Geometry check sheet. Reference: the model listing, model coordinates, mm. A direction names the side the tool comes from. Give positions to 0.01 mm unless a question says otherwise; leave off trailing zeros. Order: outer loops, then holes, each group sorted by start corner. A loop starts at its lowest first (then second) coordinate and runs counter-clockwise, first axis right, second up.
from build123d import *

# Parameters (mm, degrees)
BOSS_EXTRUDE1_DEPTH                                  = 8
CSK_FOR_M4_HEX_SOCKET_COUNTERSUNK_CAP_SC_D           = 4.5
CSK_FOR_M4_HEX_SOCKET_COUNTERSUNK_CAP_SC_CSINK_D     = 8.96
CSK_FOR_M4_HEX_SOCKET_COUNTERSUNK_CAP_SC_CSINK_ANGLE = 90
BOSS_EXTRUDE2_START                                  = -8
BOSS_EXTRUDE2_DEPTH                                  = 8
CUT_EXTRUDE1_DEPTH                                   = 6
M5_CLEARANCE_HOLE1_D                                 = 5.5


with BuildPart() as part:
    # Sketch1 → Boss-Extrude1 (new body)
    with BuildSketch(Plane.XY):
        with BuildLine():
            Line((92.897105977, 25.214321252), (49.577271028, 29.169305441))
            ThreePointArc((49.577271028, 29.169305441), (45.052575538, 34.603192698), (50.486462795, 39.127888188))
            Line((50.486462795, 39.127888188), (93.806297745, 35.172903999))
            ThreePointArc((93.806297745, 35.172903999), (98.330993235, 29.739016742), (92.897105977, 25.214321252))
        make_face()
    extrude(amount=BOSS_EXTRUDE1_DEPTH)

    # CSK for M4 Hex Socket Countersunk Cap Screw1 (through all)
    with Locations(Plane.XY.offset(8)):
        with Locations((93.351701861, 30.193612626), (50.031866911, 34.148596814)):
            CounterSinkHole(CSK_FOR_M4_HEX_SOCKET_COUNTERSUNK_CAP_SC_D / 2, CSK_FOR_M4_HEX_SOCKET_COUNTERSUNK_CAP_SC_CSINK_D / 2, counter_sink_angle=CSK_FOR_M4_HEX_SOCKET_COUNTERSUNK_CAP_SC_CSINK_ANGLE)

    # Sketch6 → Boss-Extrude2 (add)
    with BuildSketch(Plane.XY.offset(8).offset(BOSS_EXTRUDE2_START)):
        with BuildLine():
            Line((39.369723712, 30.101227002), (49.577271028, 29.169305441))
            ThreePointArc((49.577271028, 29.169305441), (45.052575538, 34.603192698), (50.486462795, 39.127888188))
            Line((50.486462795, 39.127888188), (40.278915479, 40.059809749))
            ThreePointArc((40.278915479, 40.059809749), (34.845028222, 35.535114259), (39.369723712, 30.101227002))
        make_face()
    extrude(amount=BOSS_EXTRUDE2_DEPTH)

    # Sketch8 → Cut-Extrude1 (cut)
    with BuildSketch(Plane(origin=(0, 0, 0), x_dir=(-1, 0, 0), z_dir=(0, 0, -1))):
        with BuildLine():
            Line((-39.346993918, 29.852262433), (-44.57524986, 29.374936756))
            Line((-44.57524986, 29.374936756), (-45.529901216, 39.83144864))
            Line((-45.529901216, 39.83144864), (-40.301645274, 40.308774318))
            ThreePointArc((-40.301645274, 40.308774318), (-34.596063653, 35.557844054), (-39.346993918, 29.852262433))
        make_face()
    extrude(amount=-CUT_EXTRUDE1_DEPTH, mode=Mode.SUBTRACT)

    # M5 Clearance Hole1 (through all)
    with Locations(Plane(origin=(0, 0, 6), x_dir=(-1, 0, 0), z_dir=(0, 0, -1))):
        with Locations((-39.824319596, 35.080518376)):
            Hole(M5_CLEARANCE_HOLE1_D / 2)


solid = part.part
Item 1: Sectioned sample at D-D (x = 69.5). Enter the section's corners in (y, z).
Reported:
outline: (27.35, 0) - (37.39, 0) - (37.39, 8) - (27.35, 8) - close
Item 2: Draft check along Y on faces 1 (the flat face through (45.046, 34.533, 2.958)), 2 (the cylindrical face through (37.64, 33.41, 7.01)), 3 (the flat face through (66, 33, 8)), 4 (the cylindrical face through (91.273, 29.332, 2.845)). Enter one of: released by +Y, released by -Y, zero draft, split by the parting line, or undercut.
Reported:
face 1: released by +Y
face 2: undercut
face 3: zero draft
face 4: undercut
Item 3: Sectioned sample at B-B (x = 41.5). Enter the section's corners in (y, z), and give its area (3 significant figures).
Reported:
outline: (29.91, 6) - (32.9, 6) - (32.9, 8) - (29.91, 8) - close; (37.26, 6) - (39.95, 6) - (39.95, 8) - (37.26, 8) - close
area: 11.4 mm2
Item 4: Sectioned sample at A-A (z = 3.25). Enter the section's corners in (x, y), and give its area (3 significant figures).
Reported:
outline: (44.6, 29.62) - (92.9, 25.21) arc R5 ccw to (93.81, 35.17) - (45.51, 39.58) - close; hole circle Ø4.5 at (50.03, 34.15); hole circle Ø4.5 at (93.35, 30.19)
area: 492 mm2
Item 5: Gauge pin test, flat ends, axial feed: pin 1 (1.5 mm diameter, centred on y = 33, z = 6, fed in from -X); pin 2 (3.5 mm diameter, centred on x = 50.03, y = 34.15, fed in from -Z); pin 3 (1.5 mm diameter, centred on y = 28, z = 5.5, fed in from +X); pin 4 (7 mm diameter, centred on x = 39.82, y = 35.08, fed in from -Z). Record the tip position at first contact, or that the pin passes through.
Reported:
pin 1: stops at x = 35
pin 2: passes through
pin 3: stops at x = 98.14
pin 4: stops at z = 6
Item 6: Set-up check for faces 5 (the flat face through (71, 32, 0)), 6 (the flat face through (42.5, 33.8, 6)): record each of +Z, -Z, +X, -X, +Y, -Y from which the full face is reachable in a straight line by a thin tool's end or side.
Reported:
face 5: -Z, +X, -X, +Y, -Y
face 6: -Z, -X, +Y
Item 7: Sectioned sample at C-C (y = 33.25). Give the number of separate pieces and of enclosed holes in the cut face, and give its area (3 significant figures).
Reported:
separate pieces: 3
enclosed holes: 0
area: 386 mm2
Item 8: Scan lines: L1, parallel to X at y = 32.25, z = 3.75; L2, parallel to Z at x = 42.5, y = 36; L3, parallel to X at y = 34, z = 3. Record each from-to range of solid material in increasing order.
Reported:
L1: x = 44.84 to 48.82, 51.24 to 92.44, 94.26 to 97.91
L2: z = 6 to 8
L3: x = 45 to 47.79, 52.28 to 96.59
